Autodesk Inventor part; units mm, degrees
ref_plane "YZ Plane" through (0, 0, 0) normal (1, 0, 0) x (0, 1, 0)
ref_plane "XZ Plane" through (0, 0, 0) normal (0, 1, 0) x (-1, 0, 0)
ref_plane "XY Plane" through (0, 0, 0) normal (0, 0, 1) x (1, 0, 0)
sketch "Skizze1" plane through (0, 0, 0) normal (0, 0, 1) x (1, 0, 0)
  line L0 (-15, -22.5) -> (15, -22.5)
  line L1 (15, -22.5) -> (15, 22.5)
  line L2 (15, 22.5) -> (-15, 22.5)
  line L3 (-15, 22.5) -> (-15, -22.5)
  line L4 (17.5, 25) -> (17.5, -25)
  line L5 (17.5, -25) -> (-17.5, -25)
  line L6 (-17.5, -25) -> (-17.5, 25)
  line L7 (-17.5, 25) -> (17.5, 25)
  point P0 (0, 0)
  point P1 (0, 22.5)
  point P2 (15, 0)
  dimension "d0" = 45
  dimension "d1" = 30
  dimension "d2" = 2.5
extrude "Extrusion1" add sketch "Skizze1" against normal blind 2.5 contours L3 L2 L1 L0 | L4 L5 L6 L7
extrude "Extrusion2" add sketch "Skizze1" along normal blind 77.5
sketch "Skizze2" plane through (0, 0, -2.5) normal (0, 0, -1) x (-1, 0, 0)
  circle A0 centre (0, 0) radius 1.5
  dimension "d7" = 3
extrude "Extrusion3" cut sketch "Skizze2" against normal up to surface (2.5 mm away)
sketch "Skizze3" plane through (0, 0, 77.5) normal (0, 0, 1) x (1, 0, 0)
  line L0 (5.0147, 25) -> (13.5, 25)
  line L1 (13.5, 25) -> (9.2574, 29.2426)
  line L2 (9.2574, 29.2426) -> (5.0147, 25)
  line L3 (17.5, 21) -> (17.5, 12.5147)
  line L4 (17.5, 12.5147) -> (21.7426, 16.7574)
  line L5 (21.7426, 16.7574) -> (17.5, 21)
  line L6 (17.5, 25) -> (-17.5, 25)
  line L7 (17.5, -25) -> (17.5, 25)
  line L8 (7.136, 27.1213) -> (19.6213, 14.636) construction
  line L9 (-17.5, -12.5147) -> (-17.5, -21)
  line L10 (-17.5, -21) -> (-21.7426, -16.7574)
  line L11 (-21.7426, -16.7574) -> (-17.5, -12.5147)
  line L12 (-13.5, -25) -> (-5.0147, -25)
  line L13 (-5.0147, -25) -> (-9.2574, -29.2426)
  line L14 (-9.2574, -29.2426) -> (-13.5, -25)
  line L15 (-17.5, 25) -> (-17.5, -25)
  line L16 (-17.5, -25) -> (17.5, -25)
  line L17 (-19.6213, -14.636) -> (-7.136, -27.1213) construction
  point P0 (0, 0)
  dimension "d11" = 6
  dimension "d17" = 4
  dimension "d18" = 4
extrude "Extrusion4" add sketch "Skizze3" against normal blind 6 contours L2 L1 L0 | L9 L10 L11 | L5 L4 L3 | L12 L13 L14
sketch "Skizze4" plane through (9.2574, 29.2426, 71.5) normal (-0.7071, 0.7071, 0) x (-0.7071, -0.7071, 0)
  line L0 (0, 0) -> (6, 0) construction
  line L1 (6, 6) -> (0, 6) construction
  line L2 (0, 0) -> (6, 0) construction
  line L3 (6, 0) -> (6, 6) construction
  line L4 (6, 6) -> (0, 6) construction
  line L5 (0, 6) -> (0, 0) construction
  circle A0 centre (3, 3) radius 1.65
  point P0 (27.2236, -71.5)
  point P1 (3, 6)
  point P2 (0, 3)
  dimension "d14" = 3.3
extrude "Extrusion5" cut sketch "Skizze4" against normal up to surface (17.6569 mm away)
sketch "Skizze5" plane through (-17.5, -12.5147, 71.5) normal (-0.7071, 0.7071, 0) x (-0.7071, -0.7071, 0)
  line L0 (0, 0) -> (6, 0) construction
  line L1 (0, 6) -> (6, 6) construction
  line L2 (0, 0) -> (6, 0) construction
  line L3 (6, 0) -> (6, 6) construction
  line L4 (6, 6) -> (0, 6) construction
  line L5 (0, 6) -> (0, 0) construction
  circle A0 centre (3, 3) radius 1.65
  point P0 (-21.2236, -71.5)
  point P1 (3, 6)
  point P2 (0, 3)
  dimension "d19" = 3.3
extrude "Extrusion6" cut sketch "Skizze5" against normal up to surface (17.6569 mm away)
sketch "Skizze6" plane through (0, 0, 77.5) normal (0, 0, 1) x (1, 0, 0)
  line L0 (-21.7426, -29.2426) -> (21.7426, -29.2426)
  line L1 (21.7426, -29.2426) -> (21.7426, 29.2426)
  line L2 (21.7426, 29.2426) -> (-21.7426, 29.2426)
  line L3 (-21.7426, 29.2426) -> (-21.7426, -29.2426)
  line L4 (17.5, 25) -> (13.5, 25)
  line L5 (17.5, 25) -> (-17.5, 25)
  line L6 (-17.5, 25) -> (-17.5, -25)
  line L7 (-17.5, -25) -> (17.5, -25)
  line L8 (17.5, -25) -> (17.5, 25)
  point P0 (0, 0)
  point P1 (9.2574, 29.2426)
  point P2 (21.7426, 16.7574)
  point P3 (-9.2574, -29.2426)
  point P4 (-21.7426, -16.7574)
extrude "Extrusion7" cut sketch "Skizze6" against normal up to surface (6 mm away)
equation "\"d18\" = d17"
properties part number "cage"
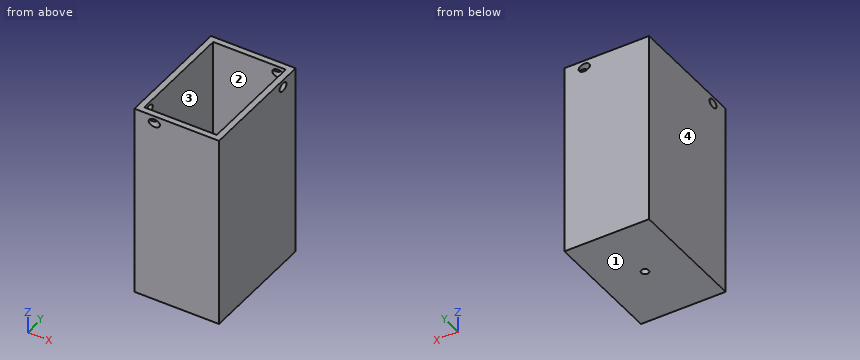
Geometry: final body of the model. Coordinates: model frame, mm. Face numbers are marked on the shaded views. Coordinates: 2 decimals unless noted, no trailing zeros. Order: outer loops, then holes, each group sorted by start corner. A loop starts at its lowest first (then second) coordinate and runs counter-clockwise, first axis right, second up. Notation, with made-up numbers: (45, -22) - (83, -22) arc R24 cw to (83, 1) - close; hole circle Ø1 at (24.5, 30.25). An arc over 180 degrees is marked (long way). Return JSON: item names as keys, results as strings. Group by question number.
1. Pull-direction query (X, two-part tool) for the marked faces 1, 2, 3 and 4; classes: pulls with the +X half, pulls with the -X half, needs draft (parallel to the pull), parting line crosses it, or undercut.
2. Pin query (flat end, axial travel): pin 1 (4 mm diameter, centred on x = 0, y = 0, fed in from +Z). Return the tip coordinate at first contact, or that it passes through.
3. Cut plane D-D (y = -5). Output: boundary loops of the cut face in (x, z).
4. Material intervals for line 1 along Y through (x, z) = (-14, 55); line 2 along X through (y, z) = (-16.5, 34); line 3 along Y through (x, z) = (0, -1.2), sorted ascending. Write a range as [from, to].
5. Cut plane B-B (x = 0). Output: boundary loops of the cut face in (y, z), plus the area to 3 significant figures.
6. Cut plane C-C (y = 0). Output: boundary loops of the cut face in (x, z).
7. Cut plane A-A (z = 44). Output: boundary loops of the cut face in (x, y).
Resolved:
{
 "1": {"face 1": "needs draft", "face 2": "undercut", "face 3": "undercut", "face 4": "pulls with the -X half"},
 "2": {"pin 1": "stops at z = 0"},
 "3": {"outline": "(-17.5, -2.5) - (17.5, -2.5) - (17.5, 77.5) - (15, 77.5) - (15, 0) - (-15, 0) - (-15, 77.5) - (-17.5, 77.5) - close"},
 "4": {"line 1": "y = [-25, -22.5], [22.5, 25]", "line 2": "x = [-17.5, -15], [15, 17.5]", "line 3": "y = [-25, -1.5], [1.5, 25]"},
 "5": {"outline": "(-25, -2.5) - (-1.5, -2.5) - (-1.5, 0) - (-22.5, 0) - (-22.5, 77.5) - (-25, 77.5) - close; (1.5, -2.5) - (25, -2.5) - (25, 77.5) - (22.5, 77.5) - (22.5, 0) - (1.5, 0) - close", "area": "505 mm²"},
 "6": {"outline": "(-17.5, -2.5) - (-1.5, -2.5) - (-1.5, 0) - (-15, 0) - (-15, 77.5) - (-17.5, 77.5) - close; (1.5, -2.5) - (17.5, -2.5) - (17.5, 77.5) - (15, 77.5) - (15, 0) - (1.5, 0) - close"},
 "7": {"outline": "(-17.5, -25) - (17.5, -25) - (17.5, 25) - (-17.5, 25) - close; hole (-15, -22.5) - (15, -22.5) - (15, 22.5) - (-15, 22.5) - close"}
}
